from build123d import *

# Parameters (mm, degrees)
SKETCH1_R           = 1.15
SKETCH1_R_2         = 0.5
BOSS_EXTRUDE1_DEPTH = 1.6
SKETCH2_R           = 1.55
SKETCH2_R_2         = 1.14
SKETCH2_R_3         = 0.9
SKETCH2_R_4         = 0.49
SKETCH2_R_5         = 1.1
BOSS_EXTRUDE2_DEPTH = 1.62
SKETCH3_R           = 3.25
BOSS_EXTRUDE3_DEPTH = 7.5


with BuildPart() as part:
    # Sketch1 → Boss-Extrude1 (new body)
    with BuildSketch(Plane(origin=(0, 0, 0), x_dir=(1, 0, 0), z_dir=(0, 1, 0))):
        with BuildLine():
            Line((-7.7, 12.25), (7.7, 12.25))
            ThreePointArc((7.7, 12.25), (9.467766953, 11.517766953), (10.2, 9.75))
            Line((10.2, 9.75), (10.2, -9.75))
            ThreePointArc((10.2, -9.75), (9.467766953, -11.517766953), (7.7, -12.25))
            Line((7.7, -12.25), (-7.7, -12.25))
            ThreePointArc((-7.7, -12.25), (-9.467766953, -11.517766953), (-10.2, -9.75))
            Line((-10.2, -9.75), (-10.2, 9.75))
            ThreePointArc((-10.2, 9.75), (-9.467766953, 11.517766953), (-7.7, 12.25))
        make_face()
        with Locations(Location((-7.7, 9.75, 0), (0, 0, 270))):
            Circle(SKETCH1_R, mode=Mode.SUBTRACT)
        with Locations(Location((7.7, 9.75, 0), (0, 0, 270))):
            Circle(SKETCH1_R, mode=Mode.SUBTRACT)
        with Locations(Location((-3.81, 9.75, 0), (0, 0, 270))):
            Circle(SKETCH1_R_2, mode=Mode.SUBTRACT)
        with Locations(Location((-1.27, 9.75, 0), (0, 0, 270))):
            Circle(SKETCH1_R_2, mode=Mode.SUBTRACT)
        with Locations(Location((1.27, 9.75, 0), (0, 0, 270))):
            Circle(SKETCH1_R_2, mode=Mode.SUBTRACT)
        with Locations(Location((3.81, 9.75, 0), (0, 0, 270))):
            Circle(SKETCH1_R_2, mode=Mode.SUBTRACT)
        with Locations(Location((-6, -8.5, 0), (0, 0, 270))):
            Circle(SKETCH1_R_2, mode=Mode.SUBTRACT)
        with Locations(Location((-2.5, -8.5, 0), (0, 0, 270))):
            Circle(SKETCH1_R_2, mode=Mode.SUBTRACT)
        with Locations(Location((6, -8.5, 0), (0, 0, 90))):
            Circle(SKETCH1_R_2, mode=Mode.SUBTRACT)
        with Locations(Location((2.5, -8.5, 0), (0, 0, 90))):
            Circle(SKETCH1_R_2, mode=Mode.SUBTRACT)
    extrude(amount=BOSS_EXTRUDE1_DEPTH)

    # Sketch2 → Boss-Extrude2 (add)
    # profile 1 of 10: a face of its own
    with BuildSketch(Plane(origin=(0, 1.61, 0), x_dir=(1, 0, 0), z_dir=(0, 1, 0))):
        with Locations(Location((7.7, 9.75, 0), (0, 0, 270))):
            Circle(SKETCH2_R)
        with Locations(Location((7.7, 9.75, 0), (0, 0, 270))):
            Circle(SKETCH2_R_2, mode=Mode.SUBTRACT)
    # profile 2 of 10: a face of its own
    with BuildSketch(Plane(origin=(0, 1.61, 0), x_dir=(1, 0, 0), z_dir=(0, 1, 0))):
        with Locations(Location((3.81, 9.75, 0), (0, 0, 270))):
            Circle(SKETCH2_R_3)
        with Locations(Location((3.81, 9.75, 0), (0, 0, 270))):
            Circle(SKETCH2_R_4, mode=Mode.SUBTRACT)
    # profile 3 of 10: a face of its own
    with BuildSketch(Plane(origin=(0, 1.61, 0), x_dir=(1, 0, 0), z_dir=(0, 1, 0))):
        with Locations(Location((1.27, 9.75, 0), (0, 0, 270))):
            Circle(SKETCH2_R_3)
        with Locations(Location((1.27, 9.75, 0), (0, 0, 270))):
            Circle(SKETCH2_R_4, mode=Mode.SUBTRACT)
    # profile 4 of 10: a face of its own
    with BuildSketch(Plane(origin=(0, 1.61, 0), x_dir=(1, 0, 0), z_dir=(0, 1, 0))):
        with Locations(Location((-1.27, 9.75, 0), (0, 0, 270))):
            Circle(SKETCH2_R_3)
        with Locations(Location((-1.27, 9.75, 0), (0, 0, 270))):
            Circle(SKETCH2_R_4, mode=Mode.SUBTRACT)
    # profile 5 of 10: a face of its own
    with BuildSketch(Plane(origin=(0, 1.61, 0), x_dir=(1, 0, 0), z_dir=(0, 1, 0))):
        with Locations(Location((-3.81, 9.75, 0), (0, 0, 270))):
            Circle(SKETCH2_R_3)
        with Locations(Location((-3.81, 9.75, 0), (0, 0, 270))):
            Circle(SKETCH2_R_4, mode=Mode.SUBTRACT)
    # profile 6 of 10: a face of its own
    with BuildSketch(Plane(origin=(0, 1.61, 0), x_dir=(1, 0, 0), z_dir=(0, 1, 0))):
        with Locations(Location((-7.7, 9.75, 0), (0, 0, 270))):
            Circle(SKETCH2_R)
        with Locations(Location((-7.7, 9.75, 0), (0, 0, 270))):
            Circle(SKETCH2_R_2, mode=Mode.SUBTRACT)
    # profile 7 of 10: a face of its own
    with BuildSketch(Plane(origin=(0, 1.61, 0), x_dir=(1, 0, 0), z_dir=(0, 1, 0))):
        with Locations(Location((-6, -8.5, 0), (0, 0, 270))):
            Circle(SKETCH2_R_5)
        with Locations(Location((-6, -8.5, 0), (0, 0, 270))):
            Circle(SKETCH2_R_4, mode=Mode.SUBTRACT)
    # profile 8 of 10: a face of its own
    with BuildSketch(Plane(origin=(0, 1.61, 0), x_dir=(1, 0, 0), z_dir=(0, 1, 0))):
        with Locations(Location((-2.5, -8.5, 0), (0, 0, 270))):
            Circle(SKETCH2_R_5)
        with Locations(Location((-2.5, -8.5, 0), (0, 0, 270))):
            Circle(SKETCH2_R_4, mode=Mode.SUBTRACT)
    # profile 9 of 10: a face of its own
    with BuildSketch(Plane(origin=(0, 1.61, 0), x_dir=(1, 0, 0), z_dir=(0, 1, 0))):
        with Locations(Location((2.5, -8.5, 0), (0, 0, 270))):
            Circle(SKETCH2_R_5)
        with Locations(Location((2.5, -8.5, 0), (0, 0, 270))):
            Circle(SKETCH2_R_4, mode=Mode.SUBTRACT)
    # profile 10 of 10: a face of its own
    with BuildSketch(Plane(origin=(0, 1.61, 0), x_dir=(1, 0, 0), z_dir=(0, 1, 0))):
        with Locations(Location((6, -8.5, 0), (0, 0, 270))):
            Circle(SKETCH2_R_5)
        with Locations(Location((6, -8.5, 0), (0, 0, 270))):
            Circle(SKETCH2_R_4, mode=Mode.SUBTRACT)
    extrude(amount=-BOSS_EXTRUDE2_DEPTH)

    # Sketch3 → Boss-Extrude3 (add)
    with BuildSketch(Plane(origin=(0, 1.6, 0), x_dir=(1, 0, 0), z_dir=(0, 1, 0))):
        with Locations(Location((-4.35038, 0.6, 0), (0, 0, 270))):
            Circle(SKETCH3_R)
    extrude(amount=BOSS_EXTRUDE3_DEPTH)


solid = part.part
The model under review builds one solid part; all positions refer to its coordinate system, in mm. Round coordinates to 2 decimals unless told otherwise and drop trailing zeros. Order: outer loops, then holes, each group sorted by start corner. A loop starts at its lowest first (then second) coordinate and runs counter-clockwise, first axis right, second up. Notation, with made-up numbers: (16, -32) -> (20, -32) arc R5 ccw to (20, -25) -> close; hole circle Ø4 at (9.5, 2). An arc over 180 degrees is marked (long way). Use CSV: the item, a comma, the result in double quotes. Start each with the question number.
(1) Insertion check: pin 1 (1.4 mm diameter, centred on x = -4, z = -10, fed in from +Y); pin 2 (0.9 mm diameter, centred on x = 8, z = -9.5, fed in from +Y); pin 3 (2 mm diameter, centred on y = 5, z = -3, fed in from -X); pin 4 (5 mm diameter, centred on x = -1, y = 2, fed in from +Z). Each pin has a flat end and moves straight along its axis. Give the tip position at first contact, or say it passes through.
(2) Mouldability with a two-part tool opening along X and no side actions: class faces 1 (the face through (6.147, 0.811, 8.967)), 2 (the face through (-9.448, 0.789, 11.537)), 3 (the face through (0, 1, 12.25)), 4 (the face through (9.448, 0.789, -11.537)) as pulls with the +X half, pulls with the -X half, needs draft (parallel to the pull), parting line crosses it, or undercut.
(3) Consider section C-C on y = 2.5. Write out the cut boundary in (x, z), and give its area (3 significant figures).
(4) Wall thickness on probe 1 along X at (y, z) = (0.9, 8.5); probe 2 along Y at (x, z) = (4.75, 9.5); probe 3 along Z at (x, y) = (-6.25, 1): over which ranges is each line inside the solid? List them lowest first. Write a range as from..to.
(5) Consider section B-B on z = 8.5. State how many separate pieces and enclosed holes the cut face has, and give its area (3 significant figures).
Responses:
1,pin 1,"y = 1.61"
1,pin 2,"through"
1,pin 3,"x = -7.28"
1,pin 4,"z = 12.25"
2,face 1,"undercut"
2,face 2,"pulls with the -X half"
2,face 3,"needs draft"
2,face 4,"pulls with the +X half"
3,outline,"circle Ø6.5 at (-4.35, -0.6)"
3,area,"33.2 mm²"
4,probe 1,"-10.2..-6.49, -5.51..-2.99, -2.01..2.01, 2.99..5.51, 6.49..10.2"
4,probe 2,"0..1.6"
4,probe 3,"-12.25..8.08, 8.92..12.25"
5,separate pieces,"5"
5,enclosed holes,"0"
5,area,"26.5 mm²"
